The model under review builds one solid part; all positions refer to its coordinate system, in mm. A direction names the side the tool comes from. Round coordinates to 2 decimals unless told otherwise and drop trailing zeros. Write each loop counter-clockwise with the first axis right and the second up, starting at its lowest first coordinate (ties: lowest second). Pieces come first, ordered by that corner, then holes. Notation, with made-up numbers: M 74,-14.75 L 133,-14.75 A16 cw 133,-3.75 Z; hole C 77,51 d11. An arc over 180 degrees is marked long. One line per item, written item: value. Start each with the question number.
1) Tool access review of faces 1 (the face through (-567, 36.1, 0)), 2 (the face through (0, 0, 25)): name each direction out of +Z, -Z, +X, -X, +Y, -Y from which nothing blocks a thin tool from reaching the whole face with its end or side.
2) Take a section at A-A, the plane y = -22.5. Write out the cut boundary in (x, z).
3) Wall thickness on probe 1 along Z at (x, y) = (-78, -34.5); probe 2 along Y at (x, z) = (-756.5, 4.5); probe 3 along Z at (x, y) = (-152, 37.35): over which ranges is each line inside the solid? List them lowest first.
4) For P1, Ø4.5, axis at x = -697, z = 0, coming from the +Y side; P2, Ø3, axis at x = -38.1, z = 0, coming from the -Y side, all flat-tipped, find the tip position at first contact; note any pin that passes through.
5) Mouldability with a two-part tool opening along Z and no side actions: class faces 3 (the face through (-567, -38.1, 0)), 4 (the face through (-567, -36.1, 0)), 5 (the face through (-567, -1, 25.4)), 6 (the face through (-567, -1, -25.4)) as +Z half, -Z half, draft (parallel to the pull), parting line (faces both ways), or undercut.
from build123d import *

# Parameters (mm, degrees)
SKETCH1_W             = 50.8
SKETCH1_H             = 76.2
BOSS_EXTRUDE1_DEPTH   = 1150
SKETCH2_W             = 46.8
SKETCH2_H             = 72.2
CUT_EXTRUDE1_DEPTH    = 1151.911278075
FILLET2_R             = 2
CROQUIS1_R            = 2.5
CORTAR_EXTRUIR1_DEPTH = 5
MATRIZL1_COUNT        = 4
MATRIZL1_PITCH        = 357.9333
CROQUIS2_R            = 2.5
CORTAR_EXTRUIR2_DEPTH = 10
CROQUIS3_R            = 2.5
CORTAR_EXTRUIR3_DEPTH = 10
CROQUIS4_R            = 2.5
CORTAR_EXTRUIR4_DEPTH = 10
MATRIZL2_COUNT        = 18
MATRIZL2_PITCH        = 60
CROQUIS5_R            = 2.5
CORTAR_EXTRUIR5_DEPTH = 10


with BuildPart() as part:
    # Sketch1 → Boss-Extrude1 (new body)
    with BuildSketch(Plane(origin=(0, 0, 0), x_dir=(0, 0, -1), z_dir=(1, 0, 0))):
        Rectangle(SKETCH1_W, SKETCH1_H)
    extrude(amount=-BOSS_EXTRUDE1_DEPTH)

    # Sketch2 → Cut-Extrude1 (cut, through all)
    with BuildSketch(Plane(origin=(0, 0, 0), x_dir=(0, 0, -1), z_dir=(1, 0, 0))):
        Rectangle(SKETCH2_W, SKETCH2_H)
    extrude(amount=-CUT_EXTRUDE1_DEPTH, mode=Mode.SUBTRACT)

    # Fillet2
    fillet2_edges = [part.edges().sort_by_distance(p)[0] for p in [
        (-575, -36.1, 23.4),
        (-575, 36.1, 23.4),
        (-575, 36.1, -23.4),
        (-575, -36.1, -23.4),
        (-575, 38.1, 25.4),
        (-575, 38.1, -25.4),
        (-575, -38.1, -25.4),
        (-575, -38.1, 25.4),
    ]]
    fillet(fillet2_edges, radius=FILLET2_R)

    # Croquis1 → Cortar-Extruir1 (cut)
    with BuildSketch(Plane.XZ.offset(38.1)):
        with Locations(Location((-38.1, 0, 0), (0, 0, 270))):
            Circle(CROQUIS1_R)
        with Locations(Location((-61.2, 15.4, 0), (0, 0, 270))):
            Circle(CROQUIS1_R)
        with Locations(Location((-15, 15.4, 0), (0, 0, 270))):
            Circle(CROQUIS1_R)
        with Locations(Location((-15, -15.4, 0), (0, 0, 270))):
            Circle(CROQUIS1_R)
        with Locations(Location((-61.2, -15.4, 0), (0, 0, 270))):
            Circle(CROQUIS1_R)
    cortar_extruir1 = extrude(amount=-CORTAR_EXTRUIR1_DEPTH, mode=Mode.SUBTRACT)

    # MatrizL1: Cortar-Extruir1 ×4
    with Locations(*[(-i * MATRIZL1_PITCH, 0, 0) for i in range(1, MATRIZL1_COUNT)]):
        add(cortar_extruir1, mode=Mode.SUBTRACT)

    # Croquis2 → Cortar-Extruir2 (cut)
    with BuildSketch(Plane.XY.offset(25.4)):
        with Locations((-225, 8.1)):
            Circle(CROQUIS2_R)
        with Locations((-1100, 8.1)):
            Circle(CROQUIS2_R)
    extrude(amount=-CORTAR_EXTRUIR2_DEPTH, mode=Mode.SUBTRACT)

    # Croquis3 → Cortar-Extruir3 (cut)
    with BuildSketch(Plane(origin=(0, 38.1, 0), x_dir=(1, 0, 0), z_dir=(0, 1, 0))):
        with Locations(Location((-152, 17.9, 0), (0, 0, 270))):
            Circle(CROQUIS3_R)
        with Locations(Location((-152, -17.9, 0), (0, 0, 270))):
            Circle(CROQUIS3_R)
        with Locations(Location((-89, -17.9, 0), (0, 0, 270))):
            Circle(CROQUIS3_R)
        with Locations(Location((-89, 17.9, 0), (0, 0, 270))):
            Circle(CROQUIS3_R)
        with Locations(Location((-31, 17.9, 0), (0, 0, 270))):
            Circle(CROQUIS3_R)
        with Locations(Location((-31, -17.9, 0), (0, 0, 270))):
            Circle(CROQUIS3_R)
    extrude(amount=-CORTAR_EXTRUIR3_DEPTH, mode=Mode.SUBTRACT)

    # Croquis4 → Cortar-Extruir4 (cut)
    with BuildSketch(Plane(origin=(0, 38.1, 0), x_dir=(1, 0, 0), z_dir=(0, 1, 0))):
        with Locations(Location((-1117, 0, 0), (0, 0, 270))):
            Circle(CROQUIS4_R)
    cortar_extruir4 = extrude(amount=-CORTAR_EXTRUIR4_DEPTH, mode=Mode.SUBTRACT)

    # MatrizL2: Cortar-Extruir4 ×18
    with Locations(*[(i * MATRIZL2_PITCH, 0, 0) for i in range(1, MATRIZL2_COUNT)]):
        add(cortar_extruir4, mode=Mode.SUBTRACT)

    # Croquis5 → Cortar-Extruir5 (cut)
    with BuildSketch(Plane(origin=(0, 38.1, 0), x_dir=(1, 0, 0), z_dir=(0, 1, 0))):
        with Locations(Location((-1121.5, 16.4, 0), (0, 0, 270))):
            Circle(CROQUIS5_R)
        with Locations(Location((-1121.5, -16.4, 0), (0, 0, 270))):
            Circle(CROQUIS5_R)
        with Locations(Location((-1139, 0, 0), (0, 0, 270))):
            Circle(CROQUIS5_R)
    extrude(amount=-CORTAR_EXTRUIR5_DEPTH, mode=Mode.SUBTRACT)


solid = part.part
Checked values:
1. face 1: +X, -X
1. face 2: +Z, -Z, +X, +Y, -Y
2. outline: M -1150,-25.4 L 0,-25.4 L 0,-23.4 L -1150,-23.4 Z; M -1150,23.4 L 0,23.4 L 0,25.4 L -1150,25.4 Z
3. probe 1: z = -25.4 to -23.36, 23.36 to 25.4
3. probe 2: y = -38.1 to -36.1, 36.1 to 38.1
3. probe 3: z = -24.96 to -20.4, -15.4 to 15.4, 20.4 to 24.96
4. P1: stops at y = -36.1
4. P2: stops at y = 36.1
5. face 3: draft
5. face 4: undercut
5. face 5: +Z half
5. face 6: -Z half
